Autodesk Inventor part; units mm, degrees
ref_plane "YZ Plane" through (0, 0, 0) normal (1, 0, 0) x (0, 1, 0)
ref_plane "XZ Plane" through (0, 0, 0) normal (0, 1, 0) x (-1, 0, 0)
ref_plane "XY Plane" through (0, 0, 0) normal (0, 0, 1) x (1, 0, 0)
sketch "Sketch1" plane through (0, 0, 0) normal (0, 0, 1) x (1, 0, 0)
  circle A0 centre (0, 0) radius 9
  dimension "d0" = 18
extrude "Extrusion1" add sketch "Sketch1" along normal blind 13.5
sketch "Sketch2" plane through (0, 0, 13.5) normal (0, 0, 1) x (1, 0, 0)
  circle A0 centre (0, 0) radius 9
  circle A1 centre (0, 0) radius 7
  dimension "d3" = 14
extrude "Extrusion2" cut sketch "Sketch2" against normal blind 11
sketch "Sketch3" plane through (0, 0, 13.5) normal (0, 0, 1) x (1, 0, 0)
  circle A0 centre (0, 0) radius 7
  circle A1 centre (0, 0) radius 5
  dimension "d6" = 10
extrude "Extrusion3" cut sketch "Sketch3" against normal blind 14 contours A1
properties part number "BUCHA DO MANCAL(41)" material "Bronze, Soft Tin"
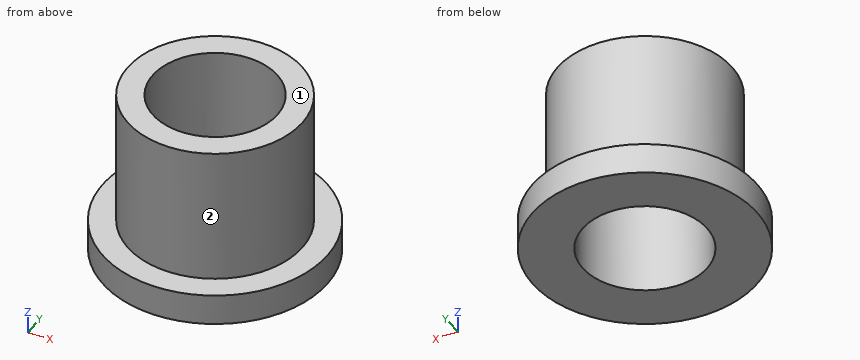
Build history of the part. All positions in model axes, mm. Face numbers are marked on the shaded views. A direction names the side the tool comes from. Give positions to 0.01 mm unless a question says otherwise; leave off trailing zeros. Loops run counter-clockwise (first coordinate to the right, second up) from the corner with the lowest first, then second, coordinate; pieces in that order, holes last. Notation, with made-up numbers: (24.5, -9.5) - (32.5, -9.5) arc R35 ccw to (32.5, 27.5) - close; hole circle Ø6 at (40, 23). An arc over 180 degrees is marked (long way). Write item = value, one per line. Start each with the question number.
1) Tool access for the marked faces 1 and 2: list every direction of +Z, -Z, +X, -X, +Y, -Y with a clear straight run to the whole face (end or side of a thin tool).
2) Band-saw the part on D-D on x = 5.5. Give the cut face in (y, z).
3) Band-saw the part on C-C on z = 4. Give the cut face in (x, y), plus the area to 3 significant figures.
4) Probe probe 1 along Y at (x, z) = (0, 10.5); probe 2 along Y at (x, z) = (-0.5, 1); probe 3 along Z at (x, y) = (-7.5, -3.5). List the from-to ranges inside material, lowest first. Write a range as from..to.
5) Drop flat-ended pins along their axis: pin 1 Ø5 at (y, z) = (1.5, 5.5) entering from -X; pin 2 Ø8 at (y, z) = (4.5, 10) entering from +X; pin 3 Ø4 at (x, z) = (-2, 6.5) entering from -Y. Give the stop position or say it passes through.
6) Band-saw the part on A-A on y = 0. Give the cut face in (x, z).
Final values:
q1.face_1 = +Z, +X, -X, +Y, -Y
q1.face_2 = +Z
q2.outline = (-7.12, 0) - (7.12, 0) - (7.12, 2.5) - (4.33, 2.5) - (4.33, 13.5) - (-4.33, 13.5) - (-4.33, 2.5) - (-7.12, 2.5) - close
q3.outline = circle Ø14 at (0, 0); hole circle Ø10 at (0, 0)
q3.area = 75.4 mm²
q4.probe_1 = -7..-5, 5..7
q4.probe_2 = -8.99..-4.97, 4.97..8.99
q4.probe_3 = 0..2.5
q5.pin_1 = -7
q5.pin_2 = 6.98
q5.pin_3 = -7
q6.outline = (-9, 0) - (-5, 0) - (-5, 13.5) - (-7, 13.5) - (-7, 2.5) - (-9, 2.5) - close; (5, 0) - (9, 0) - (9, 2.5) - (7, 2.5) - (7, 13.5) - (5, 13.5) - close
